Verification items for this drawing (mm, ordinates from the low corner). Coordinates: 2 decimals unless noted, no trailing zeros. Loops run counter-clockwise (first coordinate to the right, second up) from the corner with the lowest first, then second, coordinate; pieces in that order, holes last. Notation, with made-up numbers: M 45.25,-20 L 65.25,-20 A6 ccw 65.25,-10 Z; hole C 15,-12.5 d5. An arc over 180 degrees is marked long. Return JSON: item names as keys, results as strings.
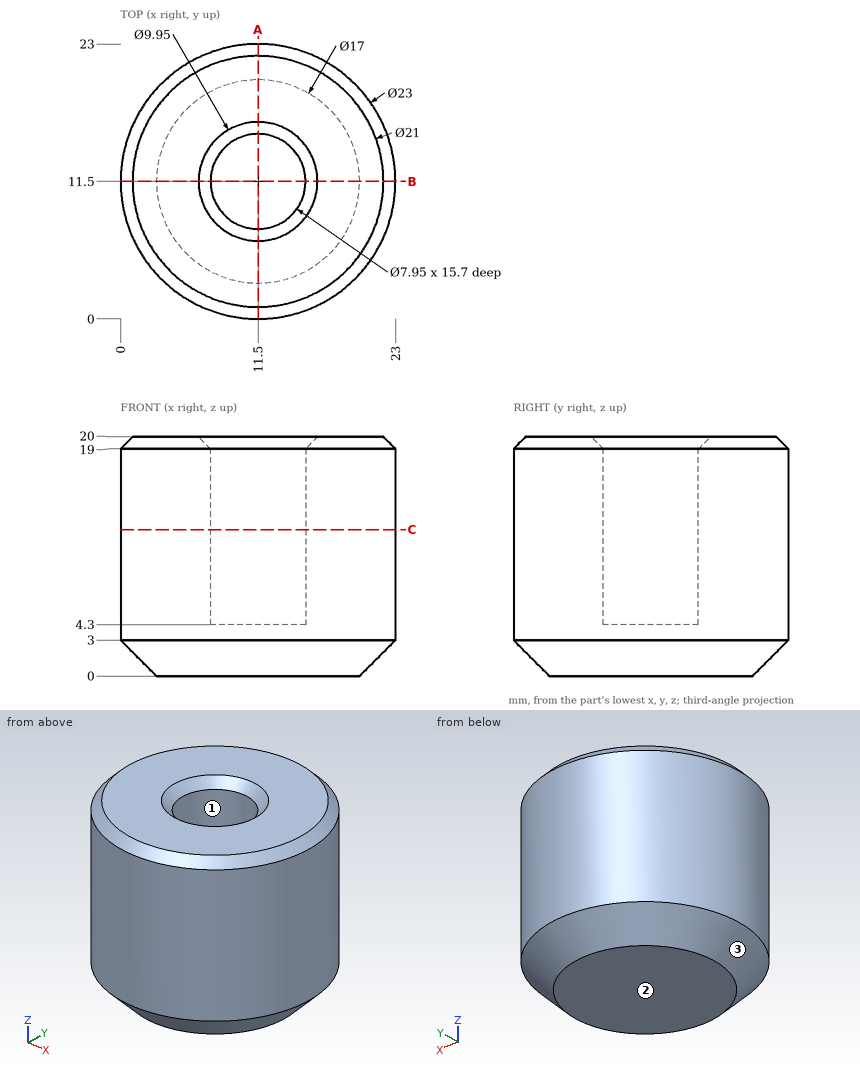
1) Section check C-C on z = 12.25. Record the cut outline in (x, y) (3 decimals).
Answers:
{"outline": "C 11.5,11.5 d23; hole C 11.5,11.5 d7.95"}
2) Scan lines: line 1 along Y through (x, z) = (11.5, 12.5) (3 decimals); line 2 along Z through (x, y) = (9, 8.75); line 3 along X through (y, z) = (12.25, 16.75). Record each from-to range of solid material in increasing order. Write a range as [from, to].
Answers:
{"line 1": "[0, 7.525], [15.475, 23]", "line 2": "[0, 4.3]", "line 3": "[0.02, 7.6], [15.4, 22.98]"}
3) Section check A-A on x = 11.5. Record the cut outline in (y, z) (3 decimals).
Answers:
{"outline": "M 0,3 L 3,0 L 20,0 L 23,3 L 23,19 L 22,20 L 16.475,20 L 15.475,19 L 15.475,4.3 L 7.525,4.3 L 7.525,19 L 6.525,20 L 1,20 L 0,19 Z"}
4) Draft check along X on the marked faces 1, 2 and 3. Enter one of: +X half, -X half, draft (parallel to the pull), parting line (faces both ways), or undercut.
Answers:
{"face 1": "undercut", "face 2": "draft", "face 3": "parting line"}
5) Go/stop test with flat-tipped pins: pin 1 Ø1 at (x, z) = (18.5, 16.5) entering from -Y; pin 2 Ø9 at (x, y) = (11.5, 11.5) entering from -Z; pin 3 Ø1.5 at (y, z) = (4, 18) entering from -X; pin 4 Ø3 at (x, y) = (10, 9) entering from +Z. Record where each tip stops, or that it passes through.
Answers:
{"pin 1": "y = 2.01", "pin 2": "z = 0", "pin 3": "x = 2.19", "pin 4": "z = 19.44"}
